Source: CAD feature listing. Evaluate the final solid. Frame: model axes, mm. Face numbers are marked on the shaded views. A direction names the side the tool comes from. Round coordinates to 2 decimals unless told otherwise and drop trailing zeros. Loops run counter-clockwise (first coordinate to the right, second up) from the corner with the lowest first, then second, coordinate; pieces in that order, holes last. Notation, with made-up numbers: (-25.5, 23.5) -> (18.5, 23.5) arc R32 cw to (18.5, 54.5) -> close; hole circle Ø1 at (36, 47.25). An arc over 180 degrees is marked (long way). Put each result on its own line as item: value. Start each with the question number.
1. Cut plane B-B (z = 13.75). Return the cut outline in (x, y), then the cut area to 3 significant figures.
2. Cut plane C-C (x = -5). Return the cut outline in (y, z), then the cut area to 3 significant figures.
3. Material intervals for L1, parallel to X at y = 12, z = 7; L2, parallel to Z at x = -25, y = -15.5; L3, parallel to Z at x = 5, y = 6.5, sorted ascending.
4. Set-up query: the marked faces 1, 2 and 3. Return all of +Z, -Z, +X, -X, +Y, -Y with unobstructed straight access to the full face (end or side cutting, diameter ignored); none if empty.
5. Contact query for flat-ended pins moving along their axis: pin 1 (13 mm diameter, centred on x = -4, y = -7, fed in from +Z); pin 2 (7.5 mm diameter, centred on y = 9.5, z = 19.5, fed in from +X); pin 3 (3 mm diameter, centred on x = -12.5, y = -15.5, fed in from +Z). Output: stop coordinate, or through.
6. Cut plane A-A (y = -4). Return the cut outline in (x, z).
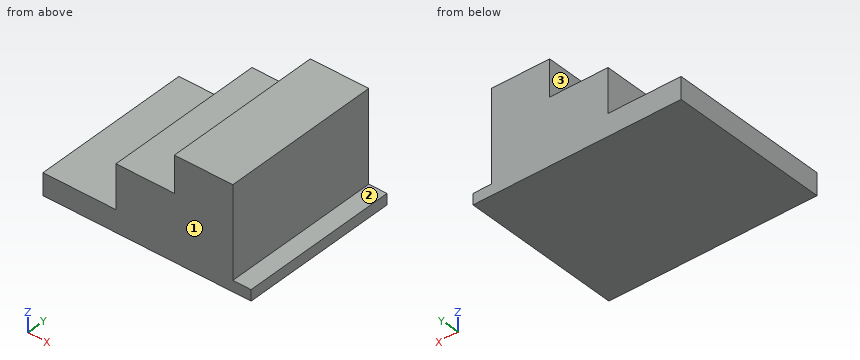
```python
from build123d import *

# Parameters (mm, degrees)
F0_W     = 57
F0_H     = 44
F1_DEPTH = 28
F2_W     = 20
F2_H     = 44
F3_DEPTH = 22
F4_W     = 16
F4_H     = 44
F5_DEPTH = 10
F6_W     = 5
F6_H     = 44
F7_DEPTH = 25


with BuildPart() as f1:
    # F0 (on Top) → F1 (new body)
    with BuildSketch(Plane.XY):
        Rectangle(F0_W, F0_H)
    extrude(amount=F1_DEPTH)

    # F2 (on face) → F3 (cut)
    with BuildSketch(Plane.XY.offset(28)):
        with Locations((-18.5, 0)):
            Rectangle(F2_W, F2_H)
    extrude(amount=-F3_DEPTH, mode=Mode.SUBTRACT)

    # F4 (on face) → F5 (cut)
    with BuildSketch(Plane.XY.offset(28)):
        with Locations((-0.5, 0)):
            Rectangle(F4_W, F4_H)
    extrude(amount=-F5_DEPTH, mode=Mode.SUBTRACT)

    # F6 (on face) → F7 (cut)
    with BuildSketch(Plane.XY.offset(28)):
        with Locations((26, 0)):
            Rectangle(F6_W, F6_H)
    extrude(amount=-F7_DEPTH, mode=Mode.SUBTRACT)


solid = f1.part
```
Solution:
1. outline: (-8.5, -22) -> (23.5, -22) -> (23.5, 22) -> (-8.5, 22) -> close
1. area: 1,410 mm^2
2. outline: (-22, 0) -> (22, 0) -> (22, 18) -> (-22, 18) -> close
2. area: 792 mm^2
3. L1: x = -8.5 to 23.5
3. L2: z = 0 to 6
3. L3: z = 0 to 18
4. face 1: +Z, -Z, +X, -X, -Y
4. face 2: +Z, +X, +Y, -Y
4. face 3: +Z, -X, +Y, -Y
5. pin 1: stops at z = 18
5. pin 2: stops at x = 23.5
5. pin 3: stops at z = 6
6. outline: (-28.5, 0) -> (28.5, 0) -> (28.5, 3) -> (23.5, 3) -> (23.5, 28) -> (7.5, 28) -> (7.5, 18) -> (-8.5, 18) -> (-8.5, 6) -> (-28.5, 6) -> close
